Could you check a few things on this drawing? It's one solid part, dimensions in mm from its lowest x, y, z. A direction names the side the tool comes from. Round coordinates to 2 decimals unless told otherwise and drop trailing zeros. Write each loop counter-clockwise with the first axis right and the second up, starting at its lowest first coordinate (ties: lowest second). Pieces come first, ordered by that corner, then holes. Notation, with made-up numbers: (-5, -15) - (6, -15) arc R28 ccw to (6, 8) - close; hole circle Ø6 at (15.5, 68). An arc over 180 degrees is marked (long way). Put each result on its own line as item: value.
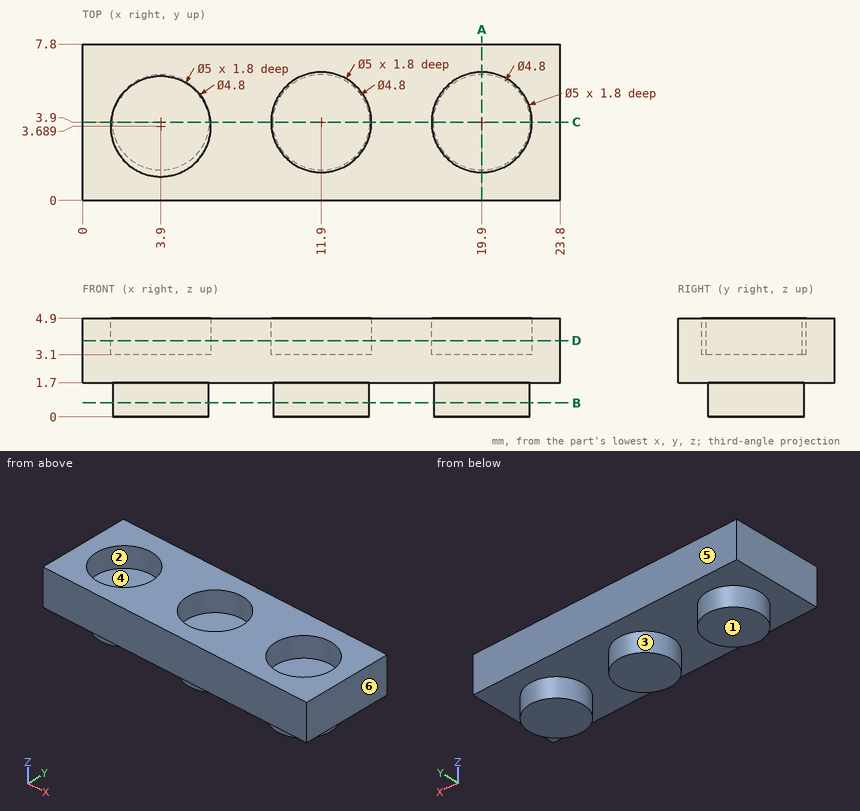
(1) Imagine slicing it at B-B, the plane z = 0.7. List the corners of the cut face in (x, y) for me, then the cut area to 3 significant figures.
Values found:
outline: circle Ø4.8 at (3.9, 3.9); circle Ø4.8 at (11.9, 3.9); circle Ø4.8 at (19.9, 3.9)
area: 54.3 mm^2
(2) I'm going to push a flat-ended pin straight in: pin 1 (3 mm diameter, centred on x = 3.9, y = 3.69, fed in from +Z). Where does the tip first touch, or does it pass through?
Values found:
pin 1: stops at z = 3.1
(3) Imagine slicing it at C-C, the plane y = 3.9. List the corners of the cut face in (x, z) for me, then the cut area to 3 significant figures.
Values found:
outline: (0, 1.7) - (1.5, 1.7) - (1.5, 0) - (6.3, 0) - (6.3, 1.7) - (9.5, 1.7) - (9.5, 0) - (14.3, 0) - (14.3, 1.7) - (17.5, 1.7) - (17.5, 0) - (22.3, 0) - (22.3, 1.7) - (23.8, 1.7) - (23.8, 4.9) - (22.4, 4.9) - (22.4, 3.1) - (17.4, 3.1) - (17.4, 4.9) - (14.4, 4.9) - (14.4, 3.1) - (9.4, 3.1) - (9.4, 4.9) - (6.39, 4.9) - (6.39, 3.1) - (1.41, 3.1) - (1.41, 4.9) - (0, 4.9) - close
area: 73.7 mm^2
(4) Please list where these lines run through material, in increasing order: probe 1 along X at (y, z) = (4.5, 4.75) (1 decimal); probe 2 along Y at (x, z) = (11.9, 4.2); probe 3 along X at (y, z) = (2, 3.6) (1 decimal). Write a range as from..to.
Values found:
probe 1: x = 0..1.5, 6.3..9.5, 14.3..17.5, 22.3..23.8
probe 2: y = 0..1.4, 6.4..7.8
probe 3: x = 0..2.1, 5.7..10.3, 13.5..18.3, 21.5..23.8
(5) Imagine slicing it at A-A, the plane x = 19.9. List the corners of the cut face in (y, z) for me.
Values found:
outline: (0, 1.7) - (1.5, 1.7) - (1.5, 0) - (6.3, 0) - (6.3, 1.7) - (7.8, 1.7) - (7.8, 4.9) - (6.4, 4.9) - (6.4, 3.1) - (1.4, 3.1) - (1.4, 4.9) - (0, 4.9) - close
(6) If we mould it in two halves opening along X, with no side actions, what happens to the marked faces 4, 5 and 6? For each: pulls with the +X half, pulls with the -X half, needs draft (parallel to the pull), parting line crosses it, or undercut.
Values found:
face 4: undercut
face 5: needs draft
face 6: pulls with the +X half
(7) Imagine slicing it at D-D, the plane z = 3.8. List the corners of the cut face in (x, y) for me.
Values found:
outline: (0, 0) - (23.8, 0) - (23.8, 7.8) - (0, 7.8) - close; hole circle Ø5 at (3.9, 3.69); hole circle Ø5 at (11.9, 3.9); hole circle Ø5 at (19.9, 3.9)
(8) For the marked faces 1, 2 and 3, which set-ups out of +Z, -Z, +X, -X, +Y, -Y let a thin tool reach every point of the face, with its end or its side?
Values found:
face 1: -Z, +X, -X, +Y, -Y
face 2: +Z
face 3: -Z
